from build123d import *

# Parameters (mm, degrees)
SALIENTE_EXTRUIR1_DEPTH = 9.525
SALIENTE_EXTRUIR2_DEPTH = 19.05
SALIENTE_EXTRUIR6_START = -82.55
CROQUIS9_W              = 19.05
CROQUIS9_H              = 19.05
CROQUIS9_W_2            = 15.875
CROQUIS9_H_2            = 15.875
SALIENTE_EXTRUIR6_DEPTH = 82.55
CROQUIS10_W             = 19.05
CROQUIS10_H             = 19.05
SALIENTE_EXTRUIR7_DEPTH = 44.45
CROQUIS11_W             = 19.05
CROQUIS11_H             = 19.05
SALIENTE_EXTRUIR8_DEPTH = 101.6
CROQUIS12_W             = 15.875
CROQUIS12_H             = 15.875
CORTAR_EXTRUIR2_DEPTH   = 565.15


with BuildPart() as part:
    # Croquis2 → Saliente-Extruir1 (new body, symmetric)
    with BuildSketch(Plane.XY):
        Polygon((-19.05, -19.05), (-19.05, 406.4), (0, 406.4), (0, 0), (444.5, 0), (444.5, -19.05), align=None)
    extrude(amount=SALIENTE_EXTRUIR1_DEPTH, both=True)



with BuildPart() as body_2:
    # Croquis3 → Saliente-Extruir2 (new body)
    with BuildSketch(Plane.XY.offset(53.975)):
        Polygon((-19.05, -19.05), (-19.05, 406.4), (0, 406.4), (0, 0), (444.5, 0), (444.5, -19.05), align=None)
    extrude(amount=SALIENTE_EXTRUIR2_DEPTH)


with BuildPart() as part_1:
    add(part.part)

    add(body_2.part)  # Saliente-Extruir6 merges body 2
    # Croquis9 → Saliente-Extruir6 (add)
    with BuildSketch(Plane.XY.offset(73.025).offset(SALIENTE_EXTRUIR6_START)):
        with Locations((-9.525, 415.925)):
            Rectangle(CROQUIS9_W, CROQUIS9_H)
        with Locations((-9.525, 415.925)):
            Rectangle(CROQUIS9_W_2, CROQUIS9_H_2, mode=Mode.SUBTRACT)
        with Locations((454.025, -9.525)):
            Rectangle(CROQUIS9_W, CROQUIS9_H)
        with Locations((454.025, -9.525)):
            Rectangle(CROQUIS9_W_2, CROQUIS9_H_2, mode=Mode.SUBTRACT)
    extrude(amount=SALIENTE_EXTRUIR6_DEPTH)

    # Croquis10 → Saliente-Extruir7 (add)
    with BuildSketch(Plane.XY.offset(9.525)):
        with Locations((-9.525, -9.525)):
            Rectangle(CROQUIS10_W, CROQUIS10_H)
    extrude(amount=SALIENTE_EXTRUIR7_DEPTH)

    # Croquis11 → Saliente-Extruir8 (add)
    with BuildSketch(Plane.ZY.offset(19.05)):
        with Locations((0, -9.525)):
            Rectangle(CROQUIS11_W, CROQUIS11_H)
        with Locations((63.5, -9.525)):
            Rectangle(CROQUIS11_W, CROQUIS11_H)
    extrude(amount=SALIENTE_EXTRUIR8_DEPTH)

    # Croquis12 → Cortar-Extruir2 (cut)
    with BuildSketch(Plane.ZY.offset(120.65)):
        with Locations((0, -9.525)):
            Rectangle(CROQUIS12_W, CROQUIS12_H)
        with Locations((63.5, -9.525)):
            Rectangle(CROQUIS12_W, CROQUIS12_H)
    extrude(amount=-CORTAR_EXTRUIR2_DEPTH, mode=Mode.SUBTRACT)


solid = part_1.part
CAD build for the part. Positions are in the model's coordinates, mm. A direction names the side the tool comes from. Coordinates: 2 decimals unless noted, no trailing zeros. Order: outer loops, then holes, each group sorted by start corner. A loop starts at its lowest first (then second) coordinate and runs counter-clockwise, first axis right, second up.
Item 1: Band-saw the part on D-D on z = 62.5. List the corners of the cut face in (x, y).
Check sheet entries:
outline: (-120.65, -19.05) - (463.55, -19.05) - (463.55, 0) - (0, 0) - (0, 425.45) - (-19.05, 425.45) - (-19.05, 0) - (-120.65, 0) - (-120.65, -1.59) - (444.5, -1.59) - (444.5, -17.46) - (-120.65, -17.46) - close; hole (-17.46, 407.99) - (-1.59, 407.99) - (-1.59, 423.86) - (-17.46, 423.86) - close; hole (446.09, -17.46) - (461.96, -17.46) - (461.96, -1.59) - (446.09, -1.59) - close
Item 2: Pin check, flat tips, straight feed: pin 1 Ø8 at (x, z) = (31.5, 0) entering from +Y; pin 2 Ø10 at (y, z) = (265.5, 56.5) entering from -X. Stop position of each tip, or through.
Check sheet entries:
pin 1: stops at y = 0
pin 2: stops at x = -19.05
Item 3: 3-axis set-ups, long thin cutter, end or side, ignore diameter. For faces 1 (the face through (-9, 206, 53.975)), 2 (the face through (-19.05, 210, 4)), 3 (the face through (454, -1.588, 31)): which of +Z, -Z, +X, -X, +Y, -Y reach the whole face in a straight line?
Check sheet entries:
face 1: +X, -X
face 2: +Z, -Z, -X, +Y
face 3: +Z, -Z
Item 4: Band-saw the part on B-B on x = 8.5. Give the number of separate pieces and of enclosed holes in the cut face, plus the area to 3 significant figures.
Check sheet entries:
separate pieces: 2
enclosed holes: 2
area: 222 mm2
Item 5: Band-saw the part on A-A on z = 22.5. List the corners of the cut face in (x, y).
Check sheet entries:
outline: (-19.05, -19.05) - (0, -19.05) - (0, 0) - (-19.05, 0) - close; (-19.05, 406.4) - (0, 406.4) - (0, 425.45) - (-19.05, 425.45) - close; (444.5, -19.05) - (463.55, -19.05) - (463.55, 0) - (444.5, 0) - close; hole (-17.46, 407.99) - (-1.59, 407.99) - (-1.59, 423.86) - (-17.46, 423.86) - close; hole (446.09, -17.46) - (461.96, -17.46) - (461.96, -1.59) - (446.09, -1.59) - close
Item 6: Drill centre lines: L1, parallel to Y at x = 244.5, z = -0.5; L2, parallel to X at y = 217.5, z = 64.5. Where is each one in solid material? Low to high.
Check sheet entries:
L1: y = -19.05 to -17.46, -1.59 to 0
L2: x = -19.05 to 0
Item 7: Two-plate mould, pull along Y, no slides. Class faces 4 (the face through (-19.05, -10, 31)), 5 (the face through (229, 0, 60)), 6 (the face through (158, -10, 55.562)), 7 (the face through (158, -1.588, 63)): +Y half, -Y half, draft (parallel to the pull), parting line (faces both ways), or undercut.
Check sheet entries:
face 4: draft
face 5: +Y half
face 6: undercut
face 7: undercut
Item 8: Band-saw the part on C-C on y = 276.5. List the corners of the cut face in (x, z) (3 decimals).
Check sheet entries:
outline: (-19.05, -9.525) - (0, -9.525) - (0, 9.525) - (-19.05, 9.525) - close; (-19.05, 53.975) - (0, 53.975) - (0, 73.025) - (-19.05, 73.025) - close
